from build123d import *

# Parameters (mm, degrees)
BOSS_EXTRU_2_DEPTH      = 6
ESQUISSE7_W             = 20
ESQUISSE7_H             = 6
ESQUISSE7_W_2           = 6
ESQUISSE7_H_2           = 15
BOSS_EXTRU_3_DEPTH      = 6
ESQUISSE8_R             = 2.5
ENL_V_MAT_EXTRU_2_DEPTH = 6


with BuildPart() as part:
    # Esquisse6 → Boss.-Extru.2 (new body)
    with BuildSketch(Plane.XY):
        Polygon((12.003078089, 22.295844579), (97.003078089, 22.295844579), (97.003078089, 7.295844579), (97.003078089, -12.704155421), (97.003078089, -27.704155421), (12.003078089, -27.704155421), (-7.996921911, -27.704155421), (-92.996921911, -27.704155421), (-92.996921911, -12.704155421), (-92.996921911, 7.295844579), (-92.996921911, 22.295844579), (-7.996921911, 22.295844579), align=None)
    extrude(amount=-BOSS_EXTRU_2_DEPTH)

    # Esquisse7 → Boss.-Extru.3 (add)
    with BuildSketch(Plane.XY):
        with Locations((2.003078089, 25.295844579)):
            Rectangle(ESQUISSE7_W, ESQUISSE7_H)
        with Locations((100.003078089, 14.795844579)):
            Rectangle(ESQUISSE7_W_2, ESQUISSE7_H_2)
        with Locations((100.003078089, -20.204155421)):
            Rectangle(ESQUISSE7_W_2, ESQUISSE7_H_2)
        with Locations((2.003078089, -30.704155421)):
            Rectangle(ESQUISSE7_W, ESQUISSE7_H)
        with Locations((-95.996921911, -20.204155421)):
            Rectangle(ESQUISSE7_W_2, ESQUISSE7_H_2)
        with Locations((-95.996921911, 14.795844579)):
            Rectangle(ESQUISSE7_W_2, ESQUISSE7_H_2)
    extrude(amount=-BOSS_EXTRU_3_DEPTH)

    # Esquisse8 → Enlèv. mat.-Extru.2 (cut)
    with BuildSketch(Plane.XY):
        with Locations((2.003078089, 18.295844579)):
            Circle(ESQUISSE8_R)
    extrude(amount=-ENL_V_MAT_EXTRU_2_DEPTH, mode=Mode.SUBTRACT)


solid = part.part
The model under review builds one solid part; all positions refer to its coordinate system, in mm. A direction names the side the tool comes from. Coordinates: 2 decimals unless noted, no trailing zeros. Write each loop counter-clockwise with the first axis right and the second up, starting at its lowest first coordinate (ties: lowest second). Pieces come first, ordered by that corner, then holes. Notation, with made-up numbers: (44.5, -7) - (86.5, -7) arc R33 cw to (86.5, 29) - close; hole circle Ø7 at (-9.75, -39). An arc over 180 degrees is marked (long way). Answer as a JSON object with one key per item and string values. Group by question number.
1. Mouldability with a two-part tool opening along Y and no side actions: class faces 4 (the face through (-53, 22.296, -3)), 5 (the face through (1.678, 20.775, -2.958)), 6 (the face through (-98.997, -20, -3)), 7 (the face through (100, -12.704, -3)) as pulls with the +Y half, pulls with the -Y half, needs draft (parallel to the pull), parting line crosses it, or undercut.
2. Clearance check with flat-ended pins moving along their axes: pin 1 Ø3 at (y, z) = (-1.5, -3) entering from +X; pin 2 Ø3 at (y, z) = (26, -2) entering from +X; pin 3 Ø3 at (y, z) = (-3, -2.5) entering from -X. State where each tip first meets the part, or that it passes through.
3. Add section B-B (x = 78.5). Give the boundary of the cut face in (y, z).
4. Machinability: for faces 1 (the face through (-7.997, 25, -3)), 2 (the face through (57, -27.704, -3)), 3 (the face through (97.003, -3, -3)), which of the approach directions +Z, -Z, +X, -X, +Y, -Y give a long, thin tool a straight path to every point of the face, cutting with its end or side? Answer none if there is none.
5. Add section C-C (y = -4.5). Give the boundary of the cut face in (x, z).
6. To check wall thickness, follow probe 1 along X at (y, z) = (-2, -0.3); probe 2 along Y at (x, z) = (-78, -1.5). State the ranges of each line that lie inside material, in increasing order.
7. Add section A-A (z = -3.7). Give the boundary of the cut face in (x, y).
Findings:
{
 "1": {"face 4": "pulls with the +Y half", "face 5": "undercut", "face 6": "needs draft", "face 7": "undercut"},
 "2": {"pin 1": "x = 97", "pin 2": "x = 12", "pin 3": "x = -93"},
 "3": {"outline": "(-27.7, -6) - (22.3, -6) - (22.3, 0) - (-27.7, 0) - close"},
 "4": {"face 1": "+Z, -Z, -X, +Y", "face 2": "+Z, -Z, +X, -Y", "face 3": "+Z, -Z, +X"},
 "5": {"outline": "(-93, -6) - (97, -6) - (97, 0) - (-93, 0) - close"},
 "6": {"probe 1": "-93 to 97", "probe 2": "-27.7 to 22.3"},
 "7": {"outline": "(-99, -27.7) - (-8, -27.7) - (-8, -33.7) - (12, -33.7) - (12, -27.7) - (103, -27.7) - (103, -12.7) - (97, -12.7) - (97, 7.3) - (103, 7.3) - (103, 22.3) - (12, 22.3) - (12, 28.3) - (-8, 28.3) - (-8, 22.3) - (-99, 22.3) - (-99, 7.3) - (-93, 7.3) - (-93, -12.7) - (-99, -12.7) - close; hole circle Ø5 at (2, 18.3)"}
}
